Check sheet for the modelled part. Datum: model origin and axes. Units: mm. A direction names the side the tool comes from. Coordinates: 2 decimals unless noted, no trailing zeros. Write each loop counter-clockwise with the first axis right and the second up, starting at its lowest first coordinate (ties: lowest second). Pieces come first, ordered by that corner, then holes. Notation, with made-up numbers: (80.5, -14.5) -> (97.5, -14.5) arc R27 cw to (97.5, 19.5) -> close; hole circle Ø9 at (6, 60). An arc over 180 degrees is marked (long way). Put each result on its own line as item: value.
```python
from build123d import *

# Parameters (mm, degrees)
SKETCH1_R           = 25
BOSS_EXTRUDE1_DEPTH = 445
SKETCH2_R           = 25
BOSS_EXTRUDE2_DEPTH = 45
CHAMFER1_SIZE       = 4


with BuildPart() as part:
    # Sketch1 → Boss-Extrude1 (new body)
    with BuildSketch(Plane(origin=(0, 0, 0), x_dir=(1, 0, 0), z_dir=(0, 1, 0))):
        with Locations(Location((0, 0, 0), (0, 0, 270))):
            Circle(SKETCH1_R)
    extrude(amount=BOSS_EXTRUDE1_DEPTH)

    # Sketch2 → Boss-Extrude2 (add)
    with BuildSketch(Plane(origin=(0, 445, 0), x_dir=(1, 0, 0), z_dir=(0, 1, 0))):
        with Locations(Location((0, 0, 0), (0, 0, 270))):
            Circle(SKETCH2_R)
        Polygon((-30.022213998, -52), (30.022213998, -52), (60.044427996, 0), (-60.044427996, 0), align=None)
        with BuildLine():
            ThreePointArc((-25, 0), (0, -25), (25, 0))
            Line((25, 0), (-25, 0))
        make_face()
        with BuildLine():
            Line((-25, 0), (25, 0))
            ThreePointArc((25, 0), (0, 25), (-25, 0))
        make_face()
        Polygon((-60.044427996, 0), (60.044427996, 0), (30.022213998, 52), (-30.022213998, 52), align=None)
    extrude(amount=BOSS_EXTRUDE2_DEPTH)

    # Chamfer1
    chamfer1_edges = [part.edges().sort_by_distance(p)[0] for p in [
        (0, 0, -25),
    ]]
    chamfer(chamfer1_edges, length=CHAMFER1_SIZE)

    # Sketch4 → Cut-Revolve1 (revolve, cut)
    with BuildSketch(Plane.XY):
        with BuildLine():
            Line((54.044427996, 490), (54.044427996, 495.946588309))
            Line((54.044427996, 495.946588309), (66.888539308, 495.946588309))
            Line((66.888539308, 495.946588309), (66.888539308, 484))
            Line((66.888539308, 484), (60.044427996, 484))
            ThreePointArc((60.044427996, 484), (58.287068683, 488.242640687), (54.044427996, 490))
        make_face()
    revolve(axis=Axis((0, 0, 0), (0, 1, 0)), mode=Mode.SUBTRACT)


solid = part.part
```
Q1. Depth check by flat-ended pin: P1, Ø5, axis at y = 392, z = 21, coming from the +X side; P2, Ø3, axis at x = -4.5, z = -33.5, coming from the -Y side; P3, Ø6, axis at x = -10, y = 295.5, coming from the +Z side. Enter the tip coordinate at first touch or a pass-through.
Recorded:
P1: stops at x = 16.82
P2: stops at y = 445
P3: stops at z = 24
Q2. Cross-section at A-A (x = 0). Record the cut outline in (y, z), plus the area to 3 significant figures.
Recorded:
outline: (0, -21) -> (4, -25) -> (445, -25) -> (445, -52) -> (490, -52) -> (490, 52) -> (445, 52) -> (445, 25) -> (4, 25) -> (0, 21) -> close
area: 26,900 mm2
Q3. Cross-section at C-C (z = 31.5). Record the cut outline in (x, y), plus the area to 3 significant figures.
Recorded:
outline: (-41.86, 445) -> (41.86, 445) -> (41.86, 490) -> (-41.86, 490) -> close
area: 3,770 mm2
Q4. Cross-section at B-B (y = 253.5). Record the cut outline in (x, z), plus the area to 3 significant figures.
Recorded:
outline: circle Ø50 at (0, 0)
area: 1,960 mm2
Q5. Material ranges on line 1 along Y through (x, z) = (33, -15.5); line 2 along X through (y, z) = (306.5, -1); line 3 along X through (y, z) = (53, -2), recorded low to high.
Recorded:
line 1: y = 445 to 490
line 2: x = -24.98 to 24.98
line 3: x = -24.92 to 24.92
Q6. Tool access check on faces 1 (the flat face through (-26, 445, -1)), 2 (the flat face through (-44.823, 467.185, -26.364)). Record the directions out of +Z, -Z, +X, -X, +Y, -Y that give a thin tool (end or side, any length) a straight path to the whole face; none if there is none.
Recorded:
face 1: -Y
face 2: -Z, -X, +Y, -Y
